```python
from build123d import *

# Parameters (mm, degrees)
F0_R     = 1.59
F0_W     = 91.44
F0_H     = 141.6
F1_DEPTH = 2.54
F3_DEPTH = 50
F5_DEPTH = 141.6
F7_DEPTH = 2


# Not quite as in the source:
# - a feature names something its author has since deleted; it is built from what else it names


with BuildPart() as f1:
    # F0 (on Top) → F1 (new body)
    with BuildSketch(Plane.XY):
        with BuildLine():
            ThreePointArc((0, 5), (1.4644660941, 1.4644660941), (5, 0))
            Line((5, 0), (25.0039321881, 0))
            ThreePointArc((25.0039321881, 0), (26.91734935, 0.3806023374), (28.5394660941, 1.4644660941))
            Line((28.5394660941, 1.4644660941), (31.3255339059, 4.2505339059))
            ThreePointArc((31.3255339059, 4.2505339059), (32.94765065, 5.3343976626), (34.8610678119, 5.715))
            Line((34.8610678119, 5.715), (160.7189321881, 5.715))
            ThreePointArc((160.7189321881, 5.715), (162.63234935, 5.3343976626), (164.2544660941, 4.2505339059))
            Line((164.2544660941, 4.2505339059), (167.0405339059, 1.4644660941))
            ThreePointArc((167.0405339059, 1.4644660941), (168.66265065, 0.3806023374), (170.5760678119, 0))
            Line((170.5760678119, 0), (190.58, 0))
            ThreePointArc((190.58, 0), (194.1155339059, 1.4644660941), (195.58, 5))
            Line((195.58, 5), (195.58, 38.1789321881))
            ThreePointArc((195.58, 38.1789321881), (195.1993976626, 40.09234935), (194.1155339059, 41.7144660941))
            Line((194.1155339059, 41.7144660941), (191.3294660941, 44.5005339059))
            ThreePointArc((191.3294660941, 44.5005339059), (190.2456023374, 46.12265065), (189.865, 48.0360678119))
            Line((189.865, 48.0360678119), (189.865, 153.8939321881))
            ThreePointArc((189.865, 153.8939321881), (190.2456023374, 155.80734935), (191.3294660941, 157.4294660941))
            Line((191.3294660941, 157.4294660941), (194.1155339059, 160.2155339059))
            ThreePointArc((194.1155339059, 160.2155339059), (195.1993976626, 161.83765065), (195.58, 163.7510678119))
            Line((195.58, 163.7510678119), (195.58, 196.93))
            ThreePointArc((195.58, 196.93), (194.1155339059, 200.4655339059), (190.58, 201.93))
            Line((190.58, 201.93), (170.5760678119, 201.93))
            ThreePointArc((170.5760678119, 201.93), (168.66265065, 201.5493976626), (167.0405339059, 200.4655339059))
            Line((167.0405339059, 200.4655339059), (164.2544660941, 197.6794660941))
            ThreePointArc((164.2544660941, 197.6794660941), (162.63234935, 196.5956023374), (160.7189321881, 196.215))
            Line((160.7189321881, 196.215), (34.8610678119, 196.215))
            ThreePointArc((34.8610678119, 196.215), (32.94765065, 196.5956023374), (31.3255339059, 197.6794660941))
            Line((31.3255339059, 197.6794660941), (28.5394660941, 200.4655339059))
            ThreePointArc((28.5394660941, 200.4655339059), (26.91734935, 201.5493976626), (25.0039321881, 201.93))
            Line((25.0039321881, 201.93), (5, 201.93))
            ThreePointArc((5, 201.93), (1.4644660941, 200.4655339059), (0, 196.93))
            Line((0, 196.93), (0, 163.7510678119))
            ThreePointArc((0, 163.7510678119), (0.3806023374, 161.83765065), (1.4644660941, 160.2155339059))
            Line((1.4644660941, 160.2155339059), (4.2505339059, 157.4294660941))
            ThreePointArc((4.2505339059, 157.4294660941), (5.3343976626, 155.80734935), (5.715, 153.8939321881))
            Line((5.715, 153.8939321881), (5.715, 48.0360678119))
            ThreePointArc((5.715, 48.0360678119), (5.3343976626, 46.12265065), (4.2505339059, 44.5005339059))
            Line((4.2505339059, 44.5005339059), (1.4644660941, 41.7144660941))
            ThreePointArc((1.4644660941, 41.7144660941), (0.3806023374, 40.09234935), (0, 38.1789321881))
            Line((0, 38.1789321881), (0, 5))
        make_face()
        with Locations((19.05, 3.175)):
            Circle(F0_R, mode=Mode.SUBTRACT)
        with Locations((5.715, 15.875)):
            Circle(F0_R, mode=Mode.SUBTRACT)
        with Locations((5.715, 28.575)):
            Circle(F0_R, mode=Mode.SUBTRACT)
        with Locations((3.175, 37.465)):
            Circle(F0_R, mode=Mode.SUBTRACT)
        with Locations((97.79, 100.965)):
            Rectangle(F0_W, F0_H, mode=Mode.SUBTRACT)
        with Locations((176.53, 3.175)):
            Circle(F0_R, mode=Mode.SUBTRACT)
        with Locations((189.865, 15.875)):
            Circle(F0_R, mode=Mode.SUBTRACT)
        with Locations((189.865, 28.575)):
            Circle(F0_R, mode=Mode.SUBTRACT)
        with Locations((192.405, 37.465)):
            Circle(F0_R, mode=Mode.SUBTRACT)
        with Locations((3.175, 164.465)):
            Circle(F0_R, mode=Mode.SUBTRACT)
        with Locations((5.715, 173.355)):
            Circle(F0_R, mode=Mode.SUBTRACT)
        with Locations((5.715, 186.055)):
            Circle(F0_R, mode=Mode.SUBTRACT)
        with Locations((19.05, 198.755)):
            Circle(F0_R, mode=Mode.SUBTRACT)
        with Locations((192.405, 164.465)):
            Circle(F0_R, mode=Mode.SUBTRACT)
        with Locations((189.865, 173.355)):
            Circle(F0_R, mode=Mode.SUBTRACT)
        with Locations((189.865, 186.055)):
            Circle(F0_R, mode=Mode.SUBTRACT)
        with Locations((176.53, 198.755)):
            Circle(F0_R, mode=Mode.SUBTRACT)
    extrude(amount=F1_DEPTH)

    # F2 (on face) → F3 (join)
    with BuildSketch(Plane.XY.offset(2.54)):
        Polygon((9, 192.93), (9, 171.765), (52.07, 171.765), (143.51, 171.765), (186.58, 171.765), (186.58, 192.93), align=None)
        Polygon((143.51, 30.165), (52.07, 30.165), (9, 30.165), (9, 9), (186.58, 9), (186.58, 30.165), align=None)
    extrude(amount=F3_DEPTH)

    # F4 (on face) → F5 (join, through all)
    with BuildSketch(Plane.XZ.offset(-171.765)):
        Polygon((9, 2.54), (52.07, 2.54), (31.0637738537, 32.54), (9, 32.54), align=None)
        Polygon((143.51, 2.54), (186.58, 2.54), (186.58, 32.54), (173.51, 32.54), align=None)
    extrude(amount=F5_DEPTH)

    # F6 (on face) → F7 (join)
    with BuildSketch(Plane.XZ.offset(-171.765)):
        with BuildLine():
            Line((105.29, 33.9308214303), (105.29, 29.54))
            Line((105.29, 29.54), (110.79, 29.54))
            Line((110.79, 29.54), (111.79, 30.54))
            Line((111.79, 30.54), (168.51, 30.54))
            Line((168.51, 30.54), (168.51, 32.54))
            Line((168.51, 32.54), (110.2042135624, 32.54))
            ThreePointArc((110.2042135624, 32.54), (107.5652551286, 32.1739745962), (108.79, 34.54))
            Line((108.79, 34.54), (111.79, 34.54))
            Line((111.79, 34.54), (111.79, 36.54))
            Line((111.79, 36.54), (107.8991785697, 36.54))
            Line((107.8991785697, 36.54), (105.29, 33.9308214303))
        make_face()
        with BuildLine():
            Line((36.0637738537, 30.54), (83.79, 30.54))
            Line((83.79, 30.54), (84.79, 29.54))
            Line((84.79, 29.54), (90.29, 29.54))
            Line((90.29, 29.54), (90.29, 33.9308214303))
            Line((90.29, 33.9308214303), (87.6808214303, 36.54))
            Line((87.6808214303, 36.54), (83.79, 36.54))
            Line((83.79, 36.54), (83.79, 34.54))
            Line((83.79, 34.54), (86.79, 34.54))
            ThreePointArc((86.79, 34.54), (88.0147448714, 32.1739745962), (85.3757864376, 32.54))
            Line((85.3757864376, 32.54), (36.0637738537, 32.54))
            Line((36.0637738537, 32.54), (36.0637738537, 30.54))
        make_face()
    extrude(amount=F7_DEPTH)


solid = f1.part
```
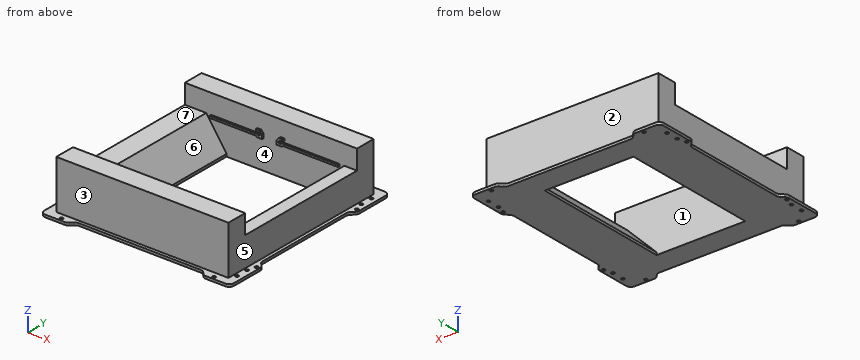
Verification items for the finished model (mm, model axes). Face numbers are marked on the shaded views. A direction names the side the tool comes from. Round coordinates to 2 decimals unless told otherwise and drop trailing zeros. Order: outer loops, then holes, each group sorted by start corner. A loop starts at its lowest first (then second) coordinate and runs counter-clockwise, first axis right, second up. Notation, with made-up numbers: (67, -2.75) - (122, -2.75) arc R31 cw to (122, 24.25) - close; hole circle Ø7 at (-16, 43). An arc over 180 degrees is marked (long way). Use CSV: the item, a comma, the result in double quotes.
(1) Section check A-A on y = 78. Record the boundary of the cut face in (x, z) (3 decimals), and give its area (3 significant figures).
Entries:
outline,"(5.715, 0) - (52.07, 0) - (52.07, 2.54) - (31.064, 32.54) - (9, 32.54) - (9, 2.54) - (5.715, 2.54) - close; (143.51, 0) - (189.865, 0) - (189.865, 2.54) - (186.58, 2.54) - (186.58, 32.54) - (173.51, 32.54) - (143.51, 2.54) - close"
area,"2,050 mm^2"
(2) Gauge pin test, flat ends, axial feed: pin 1 Ø5.5 at (x, z) = (66.5, 33) entering from -Y; pin 2 Ø1 at (y, z) = (170.5, 30.5) entering from +X; pin 3 Ø5 at (x, y) = (5.715, 186.055) entering from +Z; pin 4 Ø2.5 at (x, y) = (19.05, 3.175) entering from +Z. Record the tip position at first contact, or that the pin passes through.
Entries:
pin 1,"y = 9"
pin 2,"x = 186.58"
pin 3,"z = 2.54"
pin 4,"through"
(3) Mould release check, pull along X, two halves, no side actions. Record for the marked faces 4, 5, 6 and 7: released by +X, released by -X, zero draft, split by the parting line, or undercut.
Entries:
face 4,"undercut"
face 5,"released by +X"
face 6,"undercut"
face 7,"zero draft"
(4) Section check C-C on x = 95. Record the boundary of the cut face in (y, z) (3 decimals), and give its area (3 significant figures).
Entries:
outline,"(5.715, 0) - (30.165, 0) - (30.165, 52.54) - (9, 52.54) - (9, 2.54) - (5.715, 2.54) - close; (171.765, 0) - (196.215, 0) - (196.215, 2.54) - (192.93, 2.54) - (192.93, 52.54) - (171.765, 52.54) - close"
area,"2,240 mm^2"
(5) Section check D-D on z = 8. Record the boundary of the cut face in (x, y) (3 decimals), and give its area (3 significant figures).
Entries:
outline,"(9, 9) - (186.58, 9) - (186.58, 192.93) - (9, 192.93) - close; hole (48.247, 30.165) - (148.97, 30.165) - (148.97, 171.765) - (48.247, 171.765) - close"
area,"18,400 mm^2"
(6) Access from +Z, -Z, +X, -X, +Y, -Y to the whole of each face (thin tool, end or side, straight path). Record for the marked faces 1, 2 and 3.
Entries:
face 1,"+Z"
face 2,"+Z, +X, -X, +Y"
face 3,"+Z, +X, -X, -Y"
(7) Section check B-B on z = 39.5. Record the boundary of the cut face in (x, y) (3 decimals), and give its area (3 significant figures).
Entries:
outline,"(9, 9) - (186.58, 9) - (186.58, 30.165) - (9, 30.165) - close; (9, 171.765) - (186.58, 171.765) - (186.58, 192.93) - (9, 192.93) - close"
area,"7,520 mm^2"
(8) Thickness scan on probe 1 along Y at (x, z) = (142.5, 43) (3 decimals); probe 2 along Y at (x, z) = (122, 32.5) (3 decimals); probe 3 along Y at (x, z) = (23, 10). Record the ranges inside material, lowest first. Write a range as from..to.
Entries:
probe 1,"9..30.165, 171.765..192.93"
probe 2,"9..30.165, 169.765..192.93"
probe 3,"9..192.93"
